```python
from build123d import *

# Parameters (mm, degrees)
SKETCH_1_W          = 170
SKETCH_1_H          = 130
SKETCH_1_R          = 1.525
SKETCH_1_R_2        = 12
EXTRUDE_1_DEPTH     = 4
SKETCH_2_R          = 2.025
SKETCH_2_R_2        = 2
SKETCH_2_W          = 20
SKETCH_2_H          = 20
CUT_EXTRUDE_1_DEPTH = 4
CUT_EXTRUDE_2_DEPTH = 10
SKETCH_4_W          = 52.666666666
SKETCH_4_H          = 5
CUT_EXTRUDE_3_DEPTH = 108.079409785
FILLET_1_R          = 10


with BuildPart() as part:
    # 草图1 → 凸台-拉伸1 (new body)
    with BuildSketch(Plane(origin=(0, 0, 0), x_dir=(1, 0, 0), z_dir=(0, 1, 0))):
        Rectangle(SKETCH_1_W, SKETCH_1_H)
        with Locations(Location((0, -37, 0), (0, 0, 270))):
            Circle(SKETCH_1_R, mode=Mode.SUBTRACT)
        with Locations(Location((-32.04293994, -18.5, 0), (0, 0, 270))):
            Circle(SKETCH_1_R, mode=Mode.SUBTRACT)
        with Locations(Location((-32.04293994, 18.5, 0), (0, 0, 270))):
            Circle(SKETCH_1_R, mode=Mode.SUBTRACT)
        with Locations(Location((0, 37, 0), (0, 0, 270))):
            Circle(SKETCH_1_R, mode=Mode.SUBTRACT)
        with Locations(Location((32.04293994, 18.5, 0), (0, 0, 270))):
            Circle(SKETCH_1_R, mode=Mode.SUBTRACT)
        with Locations(Location((32.04293994, -18.5, 0), (0, 0, 270))):
            Circle(SKETCH_1_R, mode=Mode.SUBTRACT)
        with Locations(Location((0, 0, 0), (0, 0, 270))):
            Circle(SKETCH_1_R_2, mode=Mode.SUBTRACT)
    extrude(amount=EXTRUDE_1_DEPTH)

    # 草图2 → 切除-拉伸1 (cut)
    with BuildSketch(Plane(origin=(0, 4, 0), x_dir=(1, 0, 0), z_dir=(0, 1, 0))):
        with Locations(Location((-15, 60, 0), (0, 0, 270))):
            Circle(SKETCH_2_R)
        with Locations(Location((-75, 15, 0), (0, 0, 270))):
            Circle(SKETCH_2_R_2)
        with Locations(Location((75, 15, 0), (0, 0, 90))):
            Circle(SKETCH_2_R_2)
        with Locations(Location((15, 60, 0), (0, 0, 90))):
            Circle(SKETCH_2_R)
        with Locations(Location((75, -15, 0), (0, 0, 270))):
            Circle(SKETCH_2_R_2)
        with Locations(Location((-75, -15, 0), (0, 0, 90))):
            Circle(SKETCH_2_R_2)
        with Locations(Location((60, 15, 0), (0, 0, 270))):
            Circle(SKETCH_2_R)
        with Locations(Location((60, -15, 0), (0, 0, 90))):
            Circle(SKETCH_2_R)
        with Locations(Location((15, -60, 0), (0, 0, 270))):
            Circle(SKETCH_2_R)
        with Locations(Location((-15, -60, 0), (0, 0, 90))):
            Circle(SKETCH_2_R)
        with Locations(Location((-60, -15, 0), (0, 0, 270))):
            Circle(SKETCH_2_R)
        with Locations(Location((-60, 15, 0), (0, 0, 90))):
            Circle(SKETCH_2_R)
        with Locations((-75, 55)):
            Rectangle(SKETCH_2_W, SKETCH_2_H)
        with Locations((75, 55)):
            Rectangle(SKETCH_2_W, SKETCH_2_H)
        with Locations((75, -55)):
            Rectangle(SKETCH_2_W, SKETCH_2_H)
        with Locations((-75, -55)):
            Rectangle(SKETCH_2_W, SKETCH_2_H)
    extrude(amount=-CUT_EXTRUDE_1_DEPTH, mode=Mode.SUBTRACT)

    # 草图3 → 切除-拉伸2 (cut)
    with BuildSketch(Plane(origin=(0, 4, 0), x_dir=(1, 0, 0), z_dir=(0, 1, 0))):
        Polygon((-85, 20), (-85, 65), (-25, 65), align=None)
        Polygon((-85, -65), (-25, -65), (-85, -20), align=None)
        Polygon((85, -20), (85, -65), (25, -65), align=None)
        Polygon((85, 65), (25, 65), (85, 20), align=None)
    extrude(amount=-CUT_EXTRUDE_2_DEPTH, mode=Mode.SUBTRACT)

    # 草图4 → 切除-拉伸3 (cut, through all)
    with BuildSketch(Plane(origin=(0, 4, 0), x_dir=(1, 0, 0), z_dir=(0, 1, 0))):
        with Locations((0, 66.5)):
            Rectangle(SKETCH_4_W, SKETCH_4_H)
        with Locations((0, -66.5)):
            Rectangle(SKETCH_4_W, SKETCH_4_H)
    extrude(amount=-CUT_EXTRUDE_3_DEPTH, mode=Mode.SUBTRACT)

    # 圆角1
    fillet_1_edges = [part.edges().sort_by_distance(p)[0] for p in [
        (85, 2, -20),
        (85, 2, 20),
        (-85, 2, 20),
        (-85, 2, -20),
        (-26.333333333, 2, -64),
        (26.333333333, 2, -64),
        (-26.333333333, 2, 64),
        (26.333333333, 2, 64),
    ]]
    fillet(fillet_1_edges, radius=FILLET_1_R)


solid = part.part
```
Model file for the job. Use its own axes, mm. Give positions to 0.01 mm unless a question says otherwise; leave off trailing zeros. Order: outer loops, then holes, each group sorted by start corner. A loop starts at its lowest first (then second) coordinate and runs counter-clockwise, first axis right, second up.
1) Mould opens along Z. For faces 1 (the cylindrical face through (3.604, 1.972, 11.446)), 2 (the flat face through (54.6, 2, -42.8)), 3 (the flat face through (-85, 2, 0)) say: +Z half, -Z half, draft (parallel to the pull), parting line (faces both ways), or undercut.
2) Pin check, flat tips, straight feed: pin 1 (3 mm diameter, centred on x = 75, z = -15, fed in from -Y); pin 2 (1 mm diameter, centred on y = 2.5, z = 23.5, fed in from +X); pin 3 (1 mm diameter, centred on y = 2.5, z = 24, fed in from +X). Stop position of each tip, or through.
3) Saw through at C-C, the plane x = -75. Write the cut outline in (y, z).
4) Saw through at B-B, the plane x = -4. Write the cut outline in (y, z), then the cut area to 3 significant figures.
5) Saw through at A-A, the plane x = 60. Write the cut outline in (y, z) (3 decimals), then the cut area to 3 significant figures.
6) Saw through at D-D, the plane z = -52. Write the cut outline in (x, y).
7) Wall check: probe 1 along X at (y, z) = (0.8, 15) (3 decimals); probe 2 along Z at (x, y) = (-74.5, 0.3) (1 decimal); probe 3 along Z at (x, y) = (-16, 1.8). Give the ranges that are in metal, low to high.
Computed:
1. face 1: undercut
1. face 2: -Z half
1. face 3: draft
2. pin 1: passes through
2. pin 2: stops at x = 81
2. pin 3: stops at x = 80.33
3. outline: (0, -27.5) - (4, -27.5) - (4, -17) - (0, -17) - close; (0, -13) - (4, -13) - (4, 13) - (0, 13) - close; (0, 17) - (4, 17) - (4, 27.5) - (0, 27.5) - close
4. outline: (0, -64) - (4, -64) - (4, -11.31) - (0, -11.31) - close; (0, 11.31) - (4, 11.31) - (4, 64) - (0, 64) - close
4. area: 421 mm2
5. outline: (0, -38.75) - (4, -38.75) - (4, -17.025) - (0, -17.025) - close; (0, -12.975) - (4, -12.975) - (4, 12.975) - (0, 12.975) - close; (0, 17.025) - (4, 17.025) - (4, 38.75) - (0, 38.75) - close
5. area: 278 mm2
6. outline: (-42.33, 0) - (42.33, 0) - (42.33, 4) - (-42.33, 4) - close
7. probe 1: x = -85 to -77, -73 to -62.025, -57.975 to 57.975, 62.025 to 73, 77 to 85
7. probe 2: z = -27.9 to -16.9, -13.1 to 13.1, 16.9 to 27.9
7. probe 3: z = -64 to -61.76, -58.24 to 58.24, 61.76 to 64
